```python
from build123d import *

# Parameters (mm, degrees)
ESBO_O1_R                  = 3.4
RESSALTO_EXTRUS_O1_DEPTH   = 9.9
RESSALTO_EXTRUS_O1_2_DEPTH = 9.9
RESSALTO_EXTRUS_O1_3_DEPTH = 9.9
RESSALTO_EXTRUS_O1_4_DEPTH = 9.9
ESBO_O3_RX                 = 24.5
ESBO_O3_RY                 = 6.4005522
ESBO_O3_W                  = 61.1
ESBO_O3_H                  = 49
RESSALTO_EXTRUS_O2_DEPTH   = 1.26


with BuildPart() as part:
    # Esbo_o1 → Ressalto-extrus_o1 (new body)
    with BuildSketch(Plane(origin=(0, 0, 0), x_dir=(1, 0, 0), z_dir=(0, 1, 0))):
        with Locations(Location((-30.55, 30, 0), (0, 0, 90))):
            Circle(ESBO_O1_R)
    extrude(amount=RESSALTO_EXTRUS_O1_DEPTH)



with BuildPart() as body_2:
    # Esbo_o1 → Ressalto-extrus_o1 2 (new body)
    with BuildSketch(Plane(origin=(0, 0, 0), x_dir=(1, 0, 0), z_dir=(0, 1, 0))):
        with Locations(Location((-30.55, 0, 0), (0, 0, 90))):
            Circle(ESBO_O1_R)
    extrude(amount=RESSALTO_EXTRUS_O1_2_DEPTH)


with BuildPart() as body_3:
    # Esbo_o1 → Ressalto-extrus_o1 3 (new body)
    with BuildSketch(Plane(origin=(0, 0, 0), x_dir=(1, 0, 0), z_dir=(0, 1, 0))):
        with Locations(Location((30.55, 0, 0), (0, 0, 90))):
            Circle(ESBO_O1_R)
    extrude(amount=RESSALTO_EXTRUS_O1_3_DEPTH)


with BuildPart() as body_4:
    # Esbo_o1 → Ressalto-extrus_o1 4 (new body)
    with BuildSketch(Plane(origin=(0, 0, 0), x_dir=(1, 0, 0), z_dir=(0, 1, 0))):
        with Locations(Location((30.55, 30, 0), (0, 0, 90))):
            Circle(ESBO_O1_R)
    extrude(amount=RESSALTO_EXTRUS_O1_4_DEPTH)


with BuildPart() as part_1:
    add(part.part)

    add(body_2.part)  # Ressalto-extrus_o2 merges body 2

    add(body_3.part)  # Ressalto-extrus_o2 merges body 3

    add(body_4.part)  # Ressalto-extrus_o2 merges body 4
    # Esbo_o3 → Ressalto-extrus_o2 (add)
    with BuildSketch(Plane(origin=(0, 0, 0), x_dir=(1, 0, 0), z_dir=(0, 1, 0))):
        with Locations(Location((-30.55, 14.5), (0, 0, 90))):
            Ellipse(ESBO_O3_RX, ESBO_O3_RY)
        with Locations(Location((30.55, 14.5), (0, 0, 90))):
            Ellipse(ESBO_O3_RX, ESBO_O3_RY)
        with Locations((0, 14.5)):
            Rectangle(ESBO_O3_W, ESBO_O3_H)
    extrude(amount=-RESSALTO_EXTRUS_O2_DEPTH)


solid = part_1.part
```
Source: CAD feature listing. Evaluate the final solid. Frame: model axes, mm. A direction names the side the tool comes from. Coordinates: 2 decimals unless noted, no trailing zeros. Order: outer loops, then holes, each group sorted by start corner. A loop starts at its lowest first (then second) coordinate and runs counter-clockwise, first axis right, second up. Notation, with made-up numbers: (80.5, 57.25) - (105.5, 57.25) arc R17 cw to (105.5, 70.25) - close; hole circle Ø6 at (25, -1). An arc over 180 degrees is marked (long way). One line per item, written item: value.
1) Cut plane A-A on y = 7.75. Output: boundary loops of the cut face in (x, z).
Computed values:
outline: circle Ø6.8 at (-30.55, -30); circle Ø6.8 at (-30.55, 0); circle Ø6.8 at (30.55, -30); circle Ø6.8 at (30.55, 0)
2) Ray query, line 1 (Y direction, x = -16, z = -2.5); line 2 (X direction, y = 3, z = 1); line 3 (Z direction, x = 32, y = 9). Return the intervals inside material, ascending. Write a range as [from, to].
Computed values:
line 1: y = [-1.26, 0]
line 2: x = [-33.8, -27.3], [27.3, 33.8]
line 3: z = [-33.08, -26.92], [-3.08, 3.08]
3) Contact query for a flat-ended pin moving along its axis: pin 1 (2 mm diameter, centred on x = -1, z = -26.5, fed in from +Y). Output: stop coordinate, or through.
Computed values:
pin 1: stops at y = 0
4) Mould query, pull axis Z, two halves, no side actions, for faces 1 (the face through (33.87, 4.88, 0.74)), 2 (the face through (-31, 9.9, -30)). Classes: released by +Z, released by -Z, zero draft, split by the parting line, or undercut.
Computed values:
face 1: undercut
face 2: zero draft
5) Cut plane B-B on x = 10.5. Output: boundary loops of the cut face in (y, z).
Computed values:
outline: (-1.26, -39) - (0, -39) - (0, 10) - (-1.26, 10) - close
6) Reachability of faces 3 (the face through (-1, -1.26, -14)), 4 (the face through (-33.417, 4.881, -31.828)) from +Z, -Z, +X, -X, +Y, -Y: full face, straight path, thin tool, end or side. Return the list, or none.
Computed values:
face 3: +Z, -Z, +X, -X, -Y
face 4: +Y
